```python
from build123d import *
from build123d.topology import SkipClean

# Parameters (mm, degrees)
SKETCH1_R           = 1.65
BOSS_EXTRUDE1_DEPTH = 28.42
BOSS_EXTRUDE2_START = -6
BOSS_EXTRUDE2_DEPTH = 6
CUT_EXTRUDE1_DEPTH  = 448.984003326
SKETCH2_R           = 1.35
CUT_EXTRUDE2_DEPTH  = 10
CUT_EXTRUDE3_START  = -6
CUT_EXTRUDE3_DEPTH  = 2.5
SKETCH6_R           = 2.85
CUT_EXTRUDE4_DEPTH  = 25.42
CUT_EXTRUDE5_DEPTH  = 8
SKETCH9_R           = 1.25
SKETCH9_R_2         = 0.9
CUT_EXTRUDE6_DEPTH  = 3


with BuildPart() as part:
    # Sketch1 → Boss-Extrude1 (new body)
    with BuildSketch(Plane.XY):
        with BuildLine():
            Line((315.446757744, -209.334375502), (307.145931928, -204.583822928))
            ThreePointArc((307.145931928, -204.583822928), (304.839707487, -198.809610477), (309.94041472, -195.253912751))
            ThreePointArc((309.94041472, -195.253912751), (312.02997255, -194.578904366), (313.099972788, -192.661357044))
            ThreePointArc((313.099972788, -192.661357044), (316.927762492, -181.377375124), (324.717839469, -172.361005417))
            ThreePointArc((324.717839469, -172.361005417), (325.829134231, -170.467090901), (325.352638411, -168.323533116))
            ThreePointArc((325.352638411, -168.323533116), (325.834549562, -162.124503979), (331.981341697, -161.18794269))
            Line((331.981341697, -161.18794269), (340.282167513, -165.938495264))
            ThreePointArc((340.282167513, -165.938495264), (359.367624876, -169.832762492), (372.393242256, -184.315624498))
            Line((372.393242256, -184.315624498), (379.716809958, -188.506893436))
            ThreePointArc((379.716809958, -188.506893436), (382.057949767, -191.534058007), (381.572857005, -195.330022437))
            Line((381.572857005, -195.330022437), (361.70452919, -230.046726627))
            ThreePointArc((361.70452919, -230.046726627), (358.677364619, -232.387866435), (354.881400189, -231.902773674))
            Line((354.881400189, -231.902773674), (347.557832487, -227.711504736))
            ThreePointArc((347.557832487, -227.711504736), (328.472375124, -223.817237508), (315.446757744, -209.334375502))
        make_face()
        with Locations((329.49780072, -165.527530714)):
            Circle(SKETCH1_R, mode=Mode.SUBTRACT)
        with Locations((309.629472905, -200.244234904)):
            Circle(SKETCH1_R, mode=Mode.SUBTRACT)
        with Locations((357.364941166, -227.56318565)):
            Circle(SKETCH1_R, mode=Mode.SUBTRACT)
        with Locations((377.233268981, -192.84648146)):
            Circle(SKETCH1_R, mode=Mode.SUBTRACT)
        with BuildLine():
            Line((350.381017272, -175.377033761), (358.116585638, -173.27278235))
            ThreePointArc((358.116585638, -173.27278235), (370.455744319, -189.606671008), (368.091003881, -209.940356319))
            Line((368.091003881, -209.940356319), (360.355435515, -212.044607729))
            ThreePointArc((360.355435515, -212.044607729), (322.305430082, -202.70465707), (350.381017272, -175.377033761))
        make_face(mode=Mode.SUBTRACT)
    extrude(amount=BOSS_EXTRUDE1_DEPTH)

    # Sketch3 → Boss-Extrude2 (add)
    with SkipClean():  # the faces are left unmerged after this step: merging them gives an invalid solid
        with BuildSketch(Plane.XY.offset(28.42).offset(BOSS_EXTRUDE2_START)):
            with BuildLine():
                Line((350.381017272, -175.377033761), (358.116585638, -173.27278235))
                ThreePointArc((358.116585638, -173.27278235), (370.455744319, -189.606671008), (368.091003881, -209.940356319))
                Line((368.091003881, -209.940356319), (360.355435515, -212.044607729))
                ThreePointArc((360.355435515, -212.044607729), (365.534569918, -190.94534293), (350.381017272, -175.377033761))
            make_face()
        extrude(amount=BOSS_EXTRUDE2_DEPTH)

    # Sketch4 → Cut-Extrude1 (cut, through all)
    with SkipClean():  # the faces are left unmerged after this step: merging them gives an invalid solid
        with BuildSketch(Plane.XY.offset(6.02)):
            with BuildLine():
                Line((358.116585638, -173.27278235), (362.690804567, -172.028490247))
                ThreePointArc((362.690804567, -172.028490247), (368.327855438, -177.551531373), (372.393242256, -184.315624498))
                Line((372.393242256, -184.315624498), (379.716809958, -188.506893436))
                Line((379.716809958, -188.506893436), (370.706331874, -190.60065869))
                ThreePointArc((370.706331874, -190.60065869), (366.167779812, -180.660647448), (358.116585638, -173.27278235))
            make_face()
        extrude(amount=CUT_EXTRUDE1_DEPTH, mode=Mode.SUBTRACT)

    # Sketch2 → Cut-Extrude2 (cut)
    with SkipClean():  # the faces are left unmerged after this step: merging them gives an invalid solid
        with BuildSketch(Plane.XY.offset(28.42)):
            with Locations((333.892058998, -168.042359411)):
                Circle(SKETCH2_R)
            with Locations((366.872927979, -186.917270836)):
                Circle(SKETCH2_R)
            with Locations((347.004600164, -221.633975026)):
                Circle(SKETCH2_R)
            with Locations((314.023731183, -202.759063601)):
                Circle(SKETCH2_R)
        extrude(amount=-CUT_EXTRUDE2_DEPTH, mode=Mode.SUBTRACT)

    # Sketch5 → Cut-Extrude3 (cut)
    with SkipClean():  # the faces are left unmerged after this step: merging them gives an invalid solid
        with BuildSketch(Plane.XY.offset(28.42).offset(CUT_EXTRUDE3_START)):
            Polygon((347.322305423, -218.648611279), (344.578051949, -219.866152326), (344.260346689, -222.851516073), (343.72048979, -227.924360053), (348.891291479, -228.474641704), (349.431148378, -223.401797725), (349.748853638, -220.416433978), align=None)
            Polygon((317.025930942, -202.747664506), (315.514959157, -200.153382795), (312.512759397, -200.16478189), (311.021531424, -202.770462696), (309.283604434, -205.807210317), (313.796775978, -208.390092933), (315.534702968, -205.353345312), align=None)
            Polygon((332.381087213, -165.4480777), (330.889859239, -168.053758506), (332.400831025, -170.648040217), (335.403030784, -170.636641122), (336.894258757, -168.030960316), (338.632185748, -164.994212695), (334.119014203, -162.411330079), align=None)
        extrude(amount=-CUT_EXTRUDE3_DEPTH, mode=Mode.SUBTRACT)

    # Sketch6 → Cut-Extrude4 (cut)
    with SkipClean():  # the faces are left unmerged after this step: merging them gives an invalid solid
        with BuildSketch(Plane.XY.offset(28.42)):
            with Locations((309.629472905, -200.244234904)):
                Circle(SKETCH6_R)
            with Locations((329.49780072, -165.527530714)):
                Circle(SKETCH6_R)
            with Locations((357.364941166, -227.56318565)):
                Circle(SKETCH6_R)
            with Locations((377.233268981, -192.84648146)):
                Circle(SKETCH6_R)
        extrude(amount=-CUT_EXTRUDE4_DEPTH, mode=Mode.SUBTRACT)

    # Sketch7 → Cut-Extrude5 (cut)
    with SkipClean():  # the faces are left unmerged after this step: merging them gives an invalid solid
        with BuildSketch(Plane.XY.offset(28.42)):
            Polygon((314.35069552, -177.022065052), (327.846814274, -184.74587749), (333.310604423, -175.198783838), (319.814485669, -167.4749714), align=None)
            Polygon((311.867154543, -181.361653076), (325.363273297, -189.085465514), (319.899483147, -198.632559166), (306.403364394, -190.908746728), align=None)
            Polygon((362.133329989, -189.159191987), (368.208753158, -192.636149318), (379.437011765, -199.062068137), (372.48309703, -211.212914604), (361.254838422, -204.786995784), (355.179415254, -201.310038454), align=None)
        extrude(amount=-CUT_EXTRUDE5_DEPTH, mode=Mode.SUBTRACT)

    # Sketch9 → Cut-Extrude6 (cut)
    with SkipClean():  # the faces are left unmerged after this step: merging them gives an invalid solid
        with BuildSketch(Plane.XY.offset(28.42)):
            with Locations((333.590333217, -174.206689184)):
                Circle(SKETCH9_R)
            with Locations((331.502572712, -180.270619929)):
                Circle(SKETCH9_R_2)
            with Locations((328.870019276, -184.870583234)):
                Circle(SKETCH9_R_2)
            with Locations((326.388064384, -186.791494453)):
                Circle(SKETCH9_R)
            with Locations((322.661166834, -195.719553293)):
                Circle(SKETCH9_R_2)
            with Locations((319.185795551, -199.376299722)):
                Circle(SKETCH9_R)
        extrude(amount=-CUT_EXTRUDE6_DEPTH, mode=Mode.SUBTRACT)


solid = part.part
```
Here's how the part is built. I have some questions about the finished solid (model axes, mm). A direction names the side the tool comes from. Give positions to 0.01 mm unless a question says otherwise; leave off trailing zeros. Write each loop counter-clockwise with the first axis right and the second up, starting at its lowest first coordinate (ties: lowest second). Pieces come first, ordered by that corner, then holes.
(1) If I drill on L1, parallel to X at y = -198.5, z = 5.25; L2, parallel to Y at x = 344, z = 10.75; L3, parallel to Y at x = 327, z = 14.75, over which ranges is the centre line in solid material (lowest first)?
Output values:
L1: x = 304.94 to 307.38, 311.88 to 321.58, 371.37 to 379.76
L2: y = -227.92 to -219.22, -174.43 to -165.73
L3: y = -222.92 to -211.5, -182.15 to -166.9, -164.16 to -161.2
(2) Imagine slicing it at A-A, the plane z = 21.5. Count the separate pieces of the cut face and the enclosed holes in it, and give its area (3 significant figures).
Output values:
separate pieces: 5
enclosed holes: 2
area: 1,040 mm2
(3) On a 3-axis mill with a long thin cutter (end or side, diameter ignored), from which of +Z, -Z, +X, -X, +Y, -Y can I reach the whole of each face in a straight line? I mean faces 1 (the face through (366.7, -185.58, 25.46)), 2 (the face through (377, -195, 3)), 3 (the face through (332.476, -176.657, 24.476)), 4 (the face through (321, -184, 28.42)), 5 (the face through (371.263, -193.894, 8.562)). Say none if no direction works.
Output values:
face 1: +Z, -Z
face 2: +Z
face 3: +Z, -X
face 4: +Z, +X, -X, +Y, -Y
face 5: -Z
(4) Imagine slicing it at B-B, the plane x = 329. Write out the boundary of the cut face in (y, z), and give its area (3 significant figures).
Output values:
outline: (-224.11, 0) - (-213.53, 0) - (-213.53, 28.42) - (-224.11, 28.42) - close; (-180.12, 0) - (-167.1, 0) - (-167.1, 3) - (-168.33, 3) - (-168.33, 28.42) - (-172.73, 28.42) - (-172.73, 20.42) - (-180.12, 20.42) - close; (-163.95, 0) - (-160.55, 0) - (-160.55, 28.42) - (-162.72, 28.42) - (-162.72, 3) - (-163.95, 3) - close
area: 646 mm2
(5) Thinking about a two-plate mould opening in Y: for faces 6 (the face through (339, -220, 28.42)), 7 (the face through (304.814, -198.9, 14.011)), 8 (the face through (334.47, -173.32, 26.94)), which applies, pulls with the +Y half, pulls with the -Y half, needs draft (parallel to the pull), parting line crosses it, or undercut?
Output values:
face 6: needs draft
face 7: parting line crosses it
face 8: undercut
(6) Will these pins go through, and if not, where does the flat tip stop? pin 1 (4.5 mm diameter, centred on x = 309.63, y = -200.24, fed in from +Z); pin 2 (6 mm diameter, centred on y = -215, z = 8.5, fed in from +X); pin 3 (4.5 mm diameter, centred on x = 366.87, y = -186.92, fed in from -Z); pin 4 (6.5 mm diameter, centred on x = 358, y = -185.5, fed in from -Z).
Output values:
pin 1: stops at z = 3
pin 2: stops at x = 372.03
pin 3: stops at z = 22.42
pin 4: passes through
